Here's how the part is built. I have some questions about the finished solid (model axes, mm). A direction names the side the tool comes from. Coordinates: 2 decimals unless noted, no trailing zeros. Write each loop counter-clockwise with the first axis right and the second up, starting at its lowest first coordinate (ties: lowest second). Pieces come first, ordered by that corner, then holes.
Item 1: For faces 4 (the face through (125.105, -31.572, 6.877)), 5 (the face through (25, 15, 0)), 6 (the face through (25, -15, 0)), which set-ups out of +Z, -Z, +X, -X, +Y, -Y let a thin tool reach every point of the face, with its end or its side?
Item 2: I'm going to push flat-ended pins straight in: P1, Ø5, axis at x = 56.5, z = -3.5, coming from the -Y side; P2, Ø1.5, axis at x = 3.5, z = 4, coming from the +Y side; P3, Ø2, axis at y = -16.5, z = -3, coming from the -X side; P4, Ø12, axis at x = 81.5, y = -40, coming from the -Z side. Where does each tip first touch, or does it pass through?
Item 3: If we mould it in two halves opening along X, with no side actions, what happens to faces 1 (the face through (88.208, -5.915, 0.21)), 2 (the face through (-15, 0, 0)), 3 (the face through (57, -11, -15))? For each: pulls with the +X half, pulls with the -X half, needs draft (parallel to the pull), parting line crosses it, or undercut.
Item 4: I want a section at D-D (x = 61). Please give me the cut outline in (y, z), and give its area (3 significant figures).
Item 5: I want a section at A-A (z = 7). Please give me the cut outline in (x, y).
Item 6: Please list where these lines run through material, in increasing order: line 1 (Y direction, x = 27.5, z = -5.5); line 2 (X direction, y = 4.5, z = -3.5); line 3 (Y direction, x = 53.5, z = 3).
Item 7: I want a section at C-C (z = -6.75). Please give me the cut outline in (x, y), and give its area (3 significant figures).
Item 8: I want a section at B-B (x = 43). Please give me the cut outline in (y, z), and give its area (3 significant figures).
from build123d import *

# Parameters (mm, degrees)
BOSS_EXTRUDE1_DEPTH = 15
SKETCH4_R           = 12
BOSS_EXTRUDE2_DEPTH = 30
BOSS_EXTRUDE3_REACH = 169.037
SKETCH5_R           = 5


with BuildPart() as part:
    # Sketch1 → Boss-Extrude1 (new, symmetric)
    with BuildSketch(Plane.XY):
        with BuildLine():
            Line((127.5, -27.424137787), (112.5, -53.4048999))
            Line((112.5, -53.4048999), (50, -15))
            Line((50, -15), (0, -15))
            ThreePointArc((0, -15), (-15, 0), (0, 15))
            Line((0, 15), (50, 15))
            Line((50, 15), (127.5, -27.424137787))
        make_face()
    extrude(amount=BOSS_EXTRUDE1_DEPTH, both=True)

    # Sketch4 → Boss-Extrude2 (add)
    with BuildSketch(Plane(origin=(107.5, -62.065153938, 0), x_dir=(0, 0, -1), z_dir=(0.8660254037844382, -0.5000000000000008, 0))):
        with Locations(Location((0, 25, 0), (0, 0, 270))):
            Circle(SKETCH4_R)
    extrude(amount=BOSS_EXTRUDE2_DEPTH)

    # Boss-Extrude3: up to this plane
    boss_extrude3_end = Plane(origin=(122.500102159, 33.814123489, 15), z_dir=(-0.43702455737153567, -0.8994495740474913, 0))
    # Sketch5 → Boss-Extrude3 (add, up to the surface)
    with BuildSketch(Plane(origin=(17.846196254, 32.601256781, 0), x_dir=(0.877174161572964, -0.48017235475271564, 0), z_dir=(0.4801723547527156, 0.8771741615729639, 0)), mode=Mode.PRIVATE) as boss_extrude3_sk1:
        with Locations((110.008018419, 0)):
            Circle(SKETCH5_R)
    boss_extrude3_tool1 = split(extrude(boss_extrude3_sk1.sketch, amount=BOSS_EXTRUDE3_REACH, mode=Mode.PRIVATE), bisect_by=boss_extrude3_end, keep=Keep.BOTH, mode=Mode.PRIVATE)
    add(boss_extrude3_tool1.solids().sort_by_distance((114.342388, -20.221552, 0))[0])


solid = part.part
Answer:
1. face 4: none
1. face 5: +Z, -Z, -X, +Y
1. face 6: +Z, -Z, -X, -Y
2. P1: stops at y = -20.53
2. P2: stops at y = 15
2. P3: stops at x = 50.81
2. P4: stops at z = -15
3. face 1: undercut
3. face 2: pulls with the -X half
3. face 3: needs draft
4. outline: (-21.76, -15) - (8.98, -15) - (8.98, 15) - (-21.76, 15) - close
4. area: 922 mm2
5. outline: (0, -15) - (50, -15) - (112.5, -53.4) - (115.13, -48.86) - (141.11, -63.86) - (150.85, -46.97) - (124.87, -31.97) - (127.5, -27.42) - (50, 15) - (0, 15) arc R15 ccw to start
6. line 1: y = -15 to 15
6. line 2: x = -14.31 to 69.18, 123.8 to 131.95
6. line 3: y = -17.15 to 13.08
7. outline: (0, -15) - (50, -15) - (112.5, -53.4) - (115.04, -49.01) - (141.02, -64.01) - (150.94, -46.82) - (124.96, -31.82) - (127.5, -27.42) - (50, 15) - (0, 15) arc R15 ccw to start
7. area: 4,710 mm2
8. outline: (-15, -15) - (15, -15) - (15, 15) - (-15, 15) - close
8. area: 900 mm2
